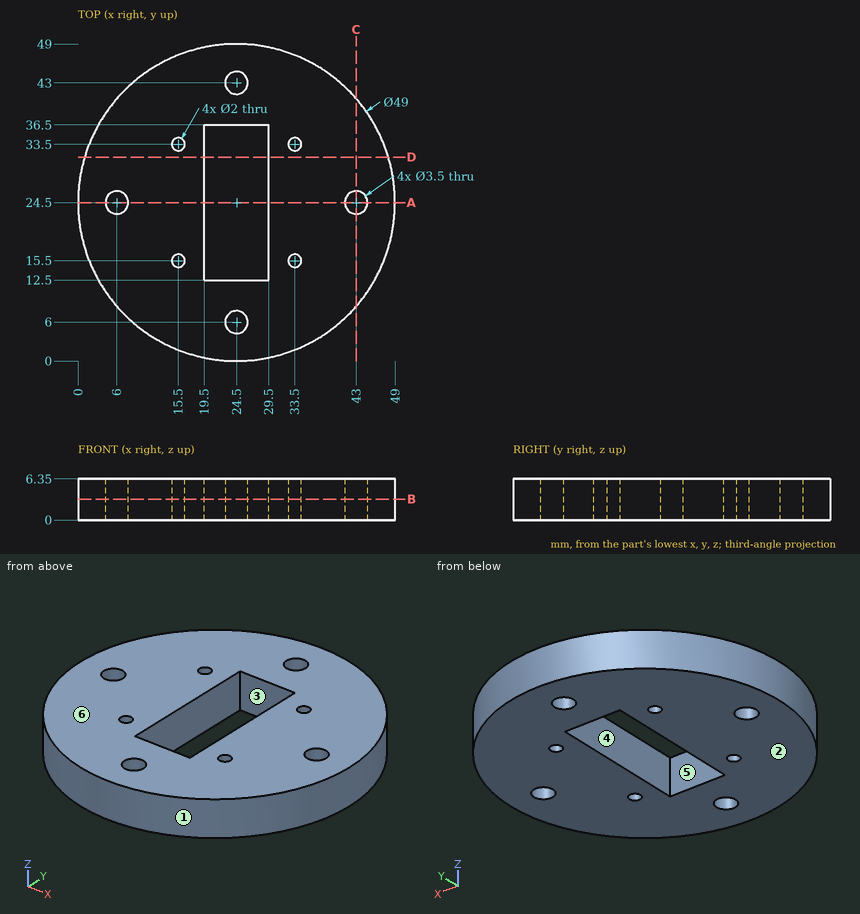
Input: dimensioned drawing with shaded views. Units: mm. Origin: part minimum x, y, z. A direction names the side the tool comes from. Give positions to 0.01 mm unless a question says otherwise; leave off trailing zeros. Order: outer loops, then holes, each group sorted by start corner. A loop starts at its lowest first (then second) coordinate and runs counter-clockwise, first axis right, second up. Notation, with made-up numbers: (-32.5, 20.5) -> (21.5, 20.5) arc R15 ccw to (21.5, 41.5) -> close; hole circle Ø10 at (15.5, -11.75). An arc over 180 degrees is marked (long way). Use a Markdown table: item, result.
1) Ray query, line 1 along Y through (x, z) = (24.5, 2.25); line 2 along X through (y, z) = (25, 5.75); line 3 along X through (y, z) = (33.5, 4.5). Return the intervals inside material, ascending. Write a range as [from, to].
Answer list:
| item | result |
|---|---|
| line 1 | [0, 4.25], [7.75, 12.5], [36.5, 41.25], [44.75, 49] |
| line 2 | [0.01, 4.32], [7.68, 19.5], [29.5, 41.32], [44.68, 48.99] |
| line 3 | [1.71, 14.5], [16.5, 19.5], [29.5, 32.5], [34.5, 47.29] |
2) Reachability of the marked faces 5 and 6 from +Z, -Z, +X, -X, +Y, -Y: full face, straight path, thin tool, end or side. Return the list, or none.
Answer list:
| item | result |
|---|---|
| face 5 | +Z, -Z |
| face 6 | +Z, +X, -X, +Y, -Y |
3) Mould query, pull axis Y, two halves, no side actions, for the marked faces 1, 2, 3 and 4. Classes: +Y half, -Y half, draft (parallel to the pull), parting line (faces both ways), or undercut.
Answer list:
| item | result |
|---|---|
| face 1 | parting line |
| face 2 | draft |
| face 3 | undercut |
| face 4 | undercut |
4) Contact query for flat-ended pins moving along their axis: P1, Ø3, axis at x = 26, z = 1.5, coming from the +Y side; P2, Ø2, axis at y = 6, z = 2, coming from the +X side; P3, Ø3, axis at x = 14.5, z = 4, coming from the -Y side. Output: stop coordinate, or through.
Answer list:
| item | result |
|---|---|
| P1 | y = 49 |
| P2 | x = 41.65 |
| P3 | y = 1.52 |
5) Section query D-D, the plane y = 31.5. Return the cut outline in (x, z).
Answer list:
| item | result |
|---|---|
| outline | (1.02, 0) -> (19.5, 0) -> (19.5, 6.35) -> (1.02, 6.35) -> close; (29.5, 0) -> (47.98, 0) -> (47.98, 6.35) -> (29.5, 6.35) -> close |
6) Section query C-C, the plane x = 43. Return the cut outline in (y, z), then the cut area to 3 significant figures.
Answer list:
| item | result |
|---|---|
| outline | (8.44, 0) -> (22.75, 0) -> (22.75, 6.35) -> (8.44, 6.35) -> close; (26.25, 0) -> (40.56, 0) -> (40.56, 6.35) -> (26.25, 6.35) -> close |
| area | 182 mm² |
7) Section query A-A, the plane y = 24.5. Return the cut outline in (x, z).
Answer list:
| item | result |
|---|---|
| outline | (0, 0) -> (4.25, 0) -> (4.25, 6.35) -> (0, 6.35) -> close; (7.75, 0) -> (19.5, 0) -> (19.5, 6.35) -> (7.75, 6.35) -> close; (29.5, 0) -> (41.25, 0) -> (41.25, 6.35) -> (29.5, 6.35) -> close; (44.75, 0) -> (49, 0) -> (49, 6.35) -> (44.75, 6.35) -> close |
8) Section query B-B, the plane z = 3.25. Count the separate pieces of the cut face and the enclosed holes in it, then the cut area to 3 significant figures.
Answer list:
| item | result |
|---|---|
| separate pieces | 1 |
| enclosed holes | 9 |
| area | 1,590 mm² |
